Source: CAD feature listing. Evaluate the final solid. Frame: model axes, mm. A direction names the side the tool comes from. Coordinates: 2 decimals unless noted, no trailing zeros. Order: outer loops, then holes, each group sorted by start corner. A loop starts at its lowest first (then second) coordinate and runs counter-clockwise, first axis right, second up.
```python
from build123d import *

# Parameters (mm, degrees)
SKETCH1_W           = 50.8
SKETCH1_H           = 50.8
BOSS_EXTRUDE1_DEPTH = 6.35
SKETCH2_R           = 10.16
SKETCH2_R_2         = 6.35
BOSS_EXTRUDE2_DEPTH = 5.08
BOSS_EXTRUDE3_DEPTH = 3.175
FILLET3_R           = 6.35
CUT_EXTRUDE1_DEPTH  = 6.35


with BuildPart() as part:
    # Sketch1 → Boss-Extrude1 (new body)
    with BuildSketch(Plane(origin=(0, 0, 0), x_dir=(1, 0, 0), z_dir=(0, 1, 0))):
        Rectangle(SKETCH1_W, SKETCH1_H)
    extrude(amount=BOSS_EXTRUDE1_DEPTH)



with BuildPart() as body_2:
    # Sketch2 → Boss-Extrude2 (new, symmetric)
    with BuildSketch(Plane.XY):
        with Locations((0, 44.45)):
            Circle(SKETCH2_R)
        with Locations((0, 44.45)):
            Circle(SKETCH2_R_2, mode=Mode.SUBTRACT)
    extrude(amount=BOSS_EXTRUDE2_DEPTH, both=True)


with BuildPart() as part_1:
    add(part.part)

    add(body_2.part)  # Boss-Extrude3 merges body 2
    # Sketch4 → Boss-Extrude3 (add, symmetric)
    with BuildSketch(Plane.XY):
        with BuildLine():
            Line((-10.16, 44.45), (-25.4, 6.35))
            Line((-25.4, 6.35), (25.4, 6.35))
            Line((25.4, 6.35), (10.16, 44.45))
            ThreePointArc((10.16, 44.45), (0, 34.29), (-10.16, 44.45))
        make_face()
    extrude(amount=BOSS_EXTRUDE3_DEPTH, both=True)

    # Fillet2: read off the stored shape, not the designer's step
    # Fillet2 outline → Fillet2 (revolve, cut)
    with BuildSketch(Plane.XZ.offset(-44.45)):
        with BuildLine():
            ThreePointArc((10.16, -3.81), (9.788025612, -4.708025612), (8.89, -5.08))
            Line((8.89, -5.08), (10.16, -5.08))
            Line((10.16, -5.08), (10.16, -3.81))
        make_face()
        with BuildLine():
            ThreePointArc((8.89, 5.08), (9.788025612, 4.708025612), (10.16, 3.81))
            Line((10.16, 3.81), (10.16, 5.08))
            Line((10.16, 5.08), (8.89, 5.08))
        make_face()
    revolve(axis=Axis((0, 44.45, 0), (0, 0, 1)), mode=Mode.SUBTRACT)

    # Fillet3
    # the kernel refuses this fillet: 6.35 mm, written as the material it adds along each edge
    with BuildSketch(Plane(origin=(10.16, 44.45, 3.175), x_dir=(-0.041343675933645734, 0.9991449847045691, 0), z_dir=(0, 0, -1))) as fillet3_piece_1:
        with BuildLine():
            CenterArc((1.102635837, 6.344570653), FILLET3_R, 250.56808401, 17.062422493)
            Line((-1.009923388, 0.356282624), (0, 0))
            ThreePointArc((0, 0), (0.420051747, 0.008686955), (0.840103495, 0))
        make_face()
    extrude(amount=6.35)
    with BuildSketch(Plane(origin=(-10.16, 44.45, 3.175), x_dir=(0.04134367593364538, 0.9991449847045691, 0), z_dir=(0, 0, -1))) as fillet3_piece_2:
        with BuildLine():
            CenterArc((1.102635837, -6.344570653), FILLET3_R, 92.369493497, 17.062422493)
            Line((-1.009923388, -0.356282624), (0, 0))
            ThreePointArc((0, 0), (0.420051747, -0.008686955), (0.840103495, 0))
        make_face()
    extrude(amount=6.35)

    # Sketch6 → Cut-Extrude1 (cut)
    with BuildSketch(Plane.XY.offset(3.175)):
        with BuildLine():
            Line((-2.490630521, 19.05), (2.490630521, 19.05))
            ThreePointArc((2.490630521, 19.05), (5.160625226, 18.231170185), (6.912500762, 16.056248096))
            Line((6.912500762, 16.056248096), (7.783333841, 13.879165397))
            ThreePointArc((7.783333841, 13.879165397), (7.464533804, 10.92000353), (4.835420347, 9.525))
            Line((4.835420347, 9.525), (-4.835420347, 9.525))
            ThreePointArc((-4.835420347, 9.525), (-7.464533804, 10.92000353), (-7.783333841, 13.879165397))
            Line((-7.783333841, 13.879165397), (-6.912500762, 16.056248096))
            ThreePointArc((-6.912500762, 16.056248096), (-5.160625226, 18.231170185), (-2.490630521, 19.05))
        make_face()
    extrude(amount=-CUT_EXTRUDE1_DEPTH, mode=Mode.SUBTRACT)


solid = part_1.part
```
1. Section query C-C on x = -16. Return loops of the section in (y, z) (3 decimals), plus the area to 3 significant figures.
Findings:
outline: (0, -25.4) - (6.35, -25.4) - (6.35, -3.175) - (29.85, -3.175) - (29.85, 3.175) - (6.35, 3.175) - (6.35, 25.4) - (0, 25.4) - close
area: 472 mm2
2. Section query A-A on x = 0. Return loops of the section in (y, z) (3 decimals).
Findings:
outline: (0, -25.4) - (6.35, -25.4) - (6.35, -3.175) - (9.525, -3.175) - (9.525, 3.175) - (6.35, 3.175) - (6.35, 25.4) - (0, 25.4) - close; (19.05, -3.175) - (34.29, -3.175) - (34.29, -3.81) arc R1.27 ccw to (35.56, -5.08) - (38.1, -5.08) - (38.1, 5.08) - (35.56, 5.08) arc R1.27 ccw to (34.29, 3.81) - (34.29, 3.175) - (19.05, 3.175) - close; (50.8, -5.08) - (53.34, -5.08) arc R1.27 ccw to (54.61, -3.81) - (54.61, 3.81) arc R1.27 ccw to (53.34, 5.08) - (50.8, 5.08) - close
3. Access query for faces 1 (the face through (-10.27, 44.37, 0.04)), 2 (the face through (-2, 51, -5.08)), 3 (the face through (0, 9.525, 0)). Directions: +Z, -Z, +X, -X, +Y, -Y. A direction counts if a zero-diameter tool reaches every point of the face in a straight line with its end or side. Return the directions, or none.
Findings:
face 1: +Z, -Z, -X, +Y
face 2: -Z, +X, -X, +Y
face 3: +Z, -Z
4. Section query B-B on y = 44.45. Return loops of the section in (x, z) (3 decimals).
Findings:
outline: (-10.252, -3.175) - (-10.16, -3.175) - (-10.16, -3.81) arc R1.27 ccw to (-8.89, -5.08) - (-6.35, -5.08) - (-6.35, 5.08) - (-8.89, 5.08) arc R1.27 ccw to (-10.16, 3.81) - (-10.16, 3.175) - (-10.252, 3.175) - close; (6.35, -5.08) - (8.89, -5.08) arc R1.27 ccw to (10.16, -3.81) - (10.16, -3.175) - (10.252, -3.175) - (10.252, 3.175) - (10.16, 3.175) - (10.16, 3.81) arc R1.27 ccw to (8.89, 5.08) - (6.35, 5.08) - close
5. Pin query (flat end, axial travel): P1, Ø5, axis at y = 32, z = -7, coming from the +X side; P2, Ø6.5, axis at x = -8.5, z = 12.5, coming from the +Y side; P3, Ø1.9, axis at x = -2, z = -1.5, coming from the +Y side; P4, Ø4, axis at x = 2.5, y = 20.5, coming from the +Z side (3 decimals). Return the tip coordinate at first contact, or that it passes through.
Findings:
P1: passes through
P2: stops at y = 6.35
P3: stops at y = 54.56
P4: stops at z = 3.175
6. Ray query, line 1 (Y direction, x = 0, z = -1.25) (3 decimals); line 2 (Y direction, x = -10.5, z = -9); line 3 (Z direction, x = 16.5, y = 11) (3 decimals). Return the intervals inside material, ascending.
Findings:
line 1: y = 0 to 9.525, 19.05 to 38.1, 50.8 to 54.61
line 2: y = 0 to 6.35
line 3: z = -3.175 to 3.175
7. Section query D-D on z = 11.5. Return loops of the section in (x, y).
Findings:
outline: (-25.4, 0) - (25.4, 0) - (25.4, 6.35) - (-25.4, 6.35) - close
8. Draft query along Y for faces 4 (the face through (10.276, 44.344, 0.044)), 5 (the face through (-25.4, 3, 0)), 6 (the face through (0, 0, 0)), 7 (the face through (0, 19.05, 0)). Return one class per face: released by +Y, released by -Y, zero draft, split by the parting line, or undercut.
Findings:
face 4: released by +Y
face 5: zero draft
face 6: released by -Y
face 7: undercut
